```python
from build123d import *

# Parameters (mm, degrees)
F0_W     = 82.55
F0_H     = 82.55
F0_R     = 1.778
F0_R_2   = 28.9941
F1_DEPTH = 6.35


# Not quite as in the source:
# - a length typed as a fraction of an inch, garbled in the dataset ("3 / 203.2 mm" for 3/8 in), is restored


with BuildPart() as f1:
    # F0 (on Top) → F1 (new body)
    with BuildSketch(Plane.XY):
        Rectangle(F0_W, F0_H)
        with Locations((-33.528, -33.528)):
            Circle(F0_R, mode=Mode.SUBTRACT)
        with Locations((-24.9936, -24.9936)):
            Circle(F0_R, mode=Mode.SUBTRACT)
        with Locations((33.528, -33.528)):
            Circle(F0_R, mode=Mode.SUBTRACT)
        with Locations((24.9936, -24.9936)):
            Circle(F0_R, mode=Mode.SUBTRACT)
        with Locations((-24.9936, 24.9936)):
            Circle(F0_R, mode=Mode.SUBTRACT)
        with Locations((-33.528, 33.528)):
            Circle(F0_R, mode=Mode.SUBTRACT)
        Circle(F0_R_2, mode=Mode.SUBTRACT)
        with Locations((24.9936, 24.9936)):
            Circle(F0_R, mode=Mode.SUBTRACT)
        with Locations((33.528, 33.528)):
            Circle(F0_R, mode=Mode.SUBTRACT)
    extrude(amount=F1_DEPTH)


solid = f1.part
```
CAD build for the part. Positions are in the model's coordinates, mm. Round coordinates to 2 decimals unless told otherwise and drop trailing zeros. Write each loop counter-clockwise with the first axis right and the second up, starting at its lowest first coordinate (ties: lowest second). Pieces come first, ordered by that corner, then holes. Notation, with made-up numbers: (56, 17) -> (108, 17) arc R14 cw to (108, 26) -> close; hole circle Ø1 at (64.25, 81.5). An arc over 180 degrees is marked (long way). Answer in a Markdown table with one row per item. Add a question column.
Item 1: Saw through at A-A, the plane y = 0. Write the cut outline in (x, z) (3 decimals).
Item 2: Mould opens along Y. For faces 1 (the face through (33.143, -35.264, 3.131)), 2 (the face through (23.683, -23.792, 3.131)), 3 (the face through (-10, 28, 0)), 4 (the face through (-1, 41.275, 3)) say: pulls with the +Y half, pulls with the -Y half, needs draft (parallel to the pull), parting line crosses it, or undercut.
Item 3: Drill centre lines: line 1 (X direction, y = -33.5, z = 4.75) (3 decimals); line 2 (Y direction, x = 23.5, z = 0.5) (3 decimals); line 3 (Y direction, x = -24, z = 4) (3 decimals). Where is each one in solid material? Low to high. Write a range as from..to.
Item 4: Saw through at C-C, the plane z = 5.25. Count the separate pieces of the cut face and the enclosed holes in it, then the cut area to 3 significant figures.
Findings below:
| question | item | result |
|---|---|---|
| 1 | outline | (-41.275, 0) -> (-28.994, 0) -> (-28.994, 6.35) -> (-41.275, 6.35) -> close; (28.994, 0) -> (41.275, 0) -> (41.275, 6.35) -> (28.994, 6.35) -> close |
| 2 | face 1 | undercut |
| 2 | face 2 | undercut |
| 2 | face 3 | needs draft |
| 2 | face 4 | pulls with the +Y half |
| 3 | line 1 | x = -41.275..-35.306, -31.75..31.75, 35.306..41.275 |
| 3 | line 2 | y = -41.275..-25.958, -24.029..-16.983, 16.983..24.029, 25.958..41.275 |
| 3 | line 3 | y = -41.275..-26.468, -23.519..-16.268, 16.268..23.519, 26.468..41.275 |
| 4 | separate pieces | 1 |
| 4 | enclosed holes | 9 |
| 4 | area | 4,090 mm^2 |
